CAD build for the part. Positions are in the model's coordinates, mm. Face numbers are marked on the shaded views. A direction names the side the tool comes from. Coordinates: 2 decimals unless noted, no trailing zeros. Loops run counter-clockwise (first coordinate to the right, second up) from the corner with the lowest first, then second, coordinate; pieces in that order, holes last.
1) Saw through at C-C, the plane z = 0.5. Write the cut outline in (x, y), and give its area (3 significant figures).
2) Saw through at B-B, the plane y = 0. Write the cut outline in (x, z), and give its area (3 significant figures).
3) Saw through at D-D, the plane z = -1.3. Write the cut outline in (x, y).
4) Pin check, flat tips, straight feed: pin 1 Ø3 at (y, z) = (6, 0) entering from -X; pin 2 Ø1.5 at (x, y) = (-7.5, 3.5) entering from -Z; pin 3 Ø2 at (x, z) = (5.5, -0.5) entering from +Y. Stop position of each tip, or through.
5) Two-plate mould, pull along Y, no slides. Class the marked faces 3, 4 and 5: +Y half, -Y half, draft (parallel to the pull), parting line (faces both ways), or undercut.
6) Saw through at A-A, the plane x = 0. Write the cut outline in (y, z).
7) Which spindle directions (+Z, -Z, +X, -X, +Y, -Y) get a long thin tool onto all of the face, cutting with end or side? Do the marked faces 1 and 2. Say none if no direction does.
8) Wall check: line 1 along Y through (x, z) = (-0.5, 0.75); line 2 along Y through (x, z) = (0, -2.15); line 3 along X through (y, z) = (4.25, 1.2). Give the ranges that are in metal, low to high.
```python
from build123d import *

# Parameters (mm, degrees)
SKETCH1_R           = 5
BOSS_EXTRUDE1_DEPTH = 4
SKETCH2_R           = 10
SKETCH2_R_2         = 1.25
BOSS_EXTRUDE2_DEPTH = 2
SKETCH3_R           = 1.5
CUT_EXTRUDE1_DEPTH  = 16.362291496
CHAMFER1_SIZE       = 0.25


with BuildPart() as part:
    # Sketch1 → Boss-Extrude1 (new body)
    with BuildSketch(Plane.XY):
        Circle(SKETCH1_R)
    extrude(amount=-BOSS_EXTRUDE1_DEPTH)

    # Sketch2 → Boss-Extrude2 (add)
    with BuildSketch(Plane.XY):
        Circle(SKETCH2_R)
        with Locations((-6.495190528, 3.75)):
            Circle(SKETCH2_R_2, mode=Mode.SUBTRACT)
        with Locations((6.495190528, 3.75)):
            Circle(SKETCH2_R_2, mode=Mode.SUBTRACT)
        with Locations((0, -7.5)):
            Circle(SKETCH2_R_2, mode=Mode.SUBTRACT)
    extrude(amount=BOSS_EXTRUDE2_DEPTH)

    # Sketch3 → Cut-Extrude1 (cut, through all)
    with BuildSketch(Plane(origin=(0, 0, -4), x_dir=(-1, 0, 0), z_dir=(0, 0, -1))):
        Circle(SKETCH3_R)
    extrude(amount=-CUT_EXTRUDE1_DEPTH, mode=Mode.SUBTRACT)

    # Chamfer1
    chamfer1_edges = [part.edges().sort_by_distance(p)[0] for p in [
        (-5, 0, 0),
        (-5, 0, -4),
        (-10, 0, 2),
        (-10, 0, 0),
    ]]
    chamfer(chamfer1_edges, length=CHAMFER1_SIZE)


solid = part.part
```
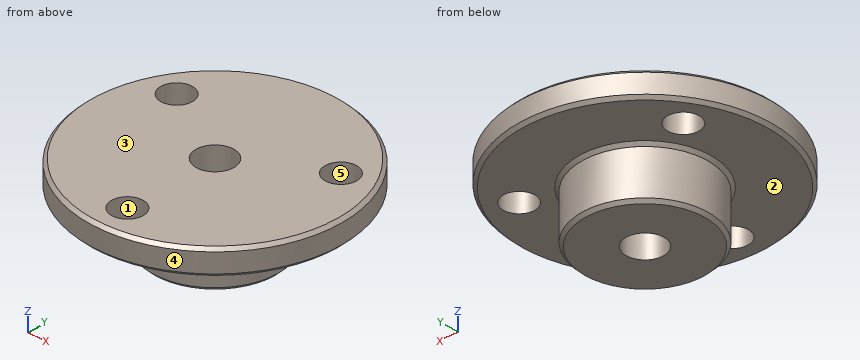
Data:
1. outline: circle Ø20 at (0, 0); hole circle Ø2.5 at (-6.5, 3.75); hole circle Ø3 at (0, 0); hole circle Ø2.5 at (0, -7.5); hole circle Ø2.5 at (6.5, 3.75)
1. area: 292 mm2
2. outline: (-10, 0.25) - (-9.75, 0) - (-5.25, 0) - (-5, -0.25) - (-5, -3.75) - (-4.75, -4) - (-1.5, -4) - (-1.5, 2) - (-9.75, 2) - (-10, 1.75) - close; (1.5, -4) - (4.75, -4) - (5, -3.75) - (5, -0.25) - (5.25, 0) - (9.75, 0) - (10, 0.25) - (10, 1.75) - (9.75, 2) - (1.5, 2) - close
2. area: 61.9 mm2
3. outline: circle Ø10 at (0, 0); hole circle Ø3 at (0, 0)
4. pin 1: stops at x = -8.92
4. pin 2: stops at z = 0
4. pin 3: stops at y = 8.75
5. face 3: draft
5. face 4: parting line
5. face 5: undercut
6. outline: (-10, 0.25) - (-9.75, 0) - (-8.75, 0) - (-8.75, 2) - (-9.75, 2) - (-10, 1.75) - close; (-6.25, 0) - (-5.25, 0) - (-5, -0.25) - (-5, -3.75) - (-4.75, -4) - (-1.5, -4) - (-1.5, 2) - (-6.25, 2) - close; (1.5, -4) - (4.75, -4) - (5, -3.75) - (5, -0.25) - (5.25, 0) - (9.75, 0) - (10, 0.25) - (10, 1.75) - (9.75, 2) - (1.5, 2) - close
7. face 1: +Z, -Z
7. face 2: -Z
8. line 1: y = -9.99 to -8.65, -6.35 to -1.41, 1.41 to 9.99
8. line 2: y = -5 to -1.5, 1.5 to 5
8. line 3: x = -9.05 to -7.64, -5.35 to 5.35, 7.64 to 9.05
